Source: CAD feature listing. Evaluate the final solid. Frame: model axes, mm. A direction names the side the tool comes from. Give positions to 0.01 mm unless a question says otherwise; leave off trailing zeros. Loops run counter-clockwise (first coordinate to the right, second up) from the corner with the lowest first, then second, coordinate; pieces in that order, holes last. Notation, with made-up numbers: (51.5, 3.5) -> (56.5, 3.5) arc R32 ccw to (56.5, 39.5) -> close; hole circle Ø5 at (79, 36). An arc over 180 degrees is marked (long way). Answer as a JSON object with one key per item and string values. Group by question number.
from build123d import *

# Parameters (mm, degrees)
SKETCH_1_R          = 2.7000000000000006
SKETCH_1_R_2        = 2.700000000000003
EXTRUDE_1_DEPTH     = 5.1
SKETCH_2_R          = 4.999999999999998
SKETCH_2_R_2        = 2.5
EXTRUDE_2_DEPTH     = 5.94
CUT_EXTRUDE_1_DEPTH = 3.5
CUT_EXTRUDE_START   = -0.6
CUT_EXTRUDE_3_DEPTH = 0.6
EXTRUDE_START       = 1.2
SKETCH_6_R          = 4.999999999999998
SKETCH_6_R_2        = 2.5
SKETCH_6_R_3        = 5
SKETCH_6_R_4        = 2.4999999999999987
EXTRUDE_4_DEPTH     = 1.2
SKETCH_7_R          = 2.6000000000000005
CUT_EXTRUDE_4_DEPTH = 33.57721194023454
SKETCH_8_R          = 2.6
CUT_EXTRUDE_5_DEPTH = 31.8406734329677
SKETCH_10_R         = 2.7
CUT_EXTRUDE_6_DEPTH = 33.57721194023454
SKETCH_11_R         = 2.700000000000001
CUT_EXTRUDE_7_DEPTH = 31.8406734329677


with BuildPart() as part:
    # Эскиз1 → Бобышка-Вытянуть1 (new body)
    with BuildSketch(Plane(origin=(0, 0, 0), x_dir=(1, 0, 0), z_dir=(0, 1, 0))):
        with BuildLine():
            Line((6.718023264525762, 8.928267668376021), (7.161238337218641, 11.37785065819786))
            Line((7.161238337218641, 11.37785065819786), (7.294846288705666, 12.560700282216452))
            Line((7.294846288705666, 12.560700282216452), (7.085001061393901, 12.665407082864023))
            Line((7.085001061393901, 12.665407082864023), (6.15987792536569, 11.916319971156167))
            Line((6.15987792536569, 11.916319971156167), (5.853623131200735, 12.10383694173367))
            Line((5.853623131200735, 12.10383694173367), (5.855060736117009, 13.29420757772634))
            Line((5.855060736117009, 13.29420757772634), (5.634886528714601, 13.37496556136943))
            Line((5.634886528714601, 13.37496556136943), (4.798663389284832, 12.527784837542624))
            Line((4.798663389284832, 12.527784837542624), (4.473480547373511, 12.680135526842204))
            Line((4.473480547373511, 12.680135526842204), (4.342730025112913, 13.863304415323501))
            Line((4.342730025112913, 13.863304415323501), (4.114949999467502, 13.919114749889351))
            Line((4.114949999467502, 13.919114749889351), (3.3779694438823102, 12.984318526945106))
            Line((3.3779694438823102, 12.984318526945106), (3.0378804853992434, 13.099618628946285))
            Line((3.0378804853992434, 13.099618628946285), (2.776558986480811, 14.260952083189514))
            Line((2.776558986480811, 14.260952083189514), (2.54399037483231, 14.291124494483034))
            Line((2.54399037483231, 14.291124494483034), (1.9153675367628848, 13.280274532718662))
            Line((1.9153675367628848, 13.280274532718662), (1.56457875493138, 13.35709799101592))
            Line((1.56457875493138, 13.35709799101592), (1.175918359734634, 14.482232389631033))
            Line((1.175918359734634, 14.482232389631033), (0.9414376205823001, 14.486393698794194))
            Line((0.9414376205823001, 14.486393698794194), (0.4289474421954887, 13.411992407470256))
            Line((0.42894744219548875, 13.411992407470256), (0.07179746795026506, 13.449389053044667))
            Line((0.07179746795026506, 13.449389053044667), (-0.4393947883485354, 14.524408492330128))
            Line((-0.43939478834853546, 14.524408492330128), (-0.6728875469021285, 14.502507231398162))
            Line((-0.6728875469021285, 14.502507231398162), (-1.062906477097084, 13.377843036257644))
            Line((-1.062906477097084, 13.377843036257644), (-1.4220003362283888, 13.375350339371238))
            Line((-1.4220003362283888, 13.375350339371238), (-2.049401918098927, 14.386958748197415))
            Line((-2.049401918098927, 14.386958748197415), (-2.279018807507275, 14.33926579666565))
            Line((-2.279018807507275, 14.33926579666565), (-2.5417426516817105, 13.178248785832608))
            Line((-2.5417426516817105, 13.178248785832608), (-2.898339045786024, 13.13589757669542))
            Line((-2.898339045786024, 13.13589757669542), (-3.6341901158202092, 14.071583165165732))
            Line((-3.6341901158202092, 14.071583165165732), (-3.8570911851181764, 13.998688399693854))
            Line((-3.8570911851181764, 13.998688399693854), (-3.989270518385492, 12.815678280718325))
            Line((-3.989270518385492, 12.815678280718325), (-4.3389589867331635, 12.733992368173748))
            Line((-4.3389589867331635, 12.733992368173748), (-5.174158380979493, 13.582182376127184))
            Line((-5.174158380979493, 13.582182376127184), (-5.3875867419063175, 13.48498737481814))
            Line((-5.3875867419063175, 13.48498737481814), (-5.3875867419063175, 12.2946158707315))
            Line((-5.3875867419063175, 12.2946158707315), (-5.751610974482103, 12.12883970299033))
            Line((-5.751610974482103, 12.12883970299033), (-6.666748566138722, 12.905854249247858))
            Line((-6.666748566138722, 12.905854249247858), (-7.13096440438616, 12.63943472468846))
            Line((-7.13096440438616, 12.63943472468846), (-7.025830916712447, 12.175864106991055))
            ThreePointArc((-7.025830916712449, 12.175864106991055), (-10.264322646127633, 9.799709596012173), (-12.51111253150909, 6.470163958468902))
            Line((-12.51111253150909, 6.470163958468902), (-5.241071220187256, 3.924995297345621))
            Line((-5.241071220187256, 3.924995297345621), (-4.737733567637334, 1.5980865565051285))
            ThreePointArc((-4.737733567637334, 1.5980865565051288), (-4.061430338102922, -2.9162962141622684), (1.55e-15, -5))
            Line((2.2e-16, -5), (21.46693589645179, -5.388260461869603))
            ThreePointArc((21.46693589645179, -5.388260461869605), (26.46693589645179, -0.3882604618696045), (21.46693589645179, 4.611739538130397))
            Line((21.46693589645179, 4.611739538130397), (7.924308406385933, 7.062073595968816))
            ThreePointArc((7.924308406385932, 7.062073595968816), (7.00463576208043, 7.790569444059032), (6.718023264525762, 8.928267668376021))
        make_face()
        with Locations(Location((21.46693589645179, -0.3882604618696027, 0), (0, 0, 270))):
            Circle(SKETCH_1_R, mode=Mode.SUBTRACT)
        with Locations(Location((-2.22e-15, -1.39e-15, 0), (0, 0, 270))):
            Circle(SKETCH_1_R_2, mode=Mode.SUBTRACT)
    extrude(amount=EXTRUDE_1_DEPTH)

    # Эскиз2 → Бобышка-Вытянуть2 (add)
    with BuildSketch(Plane(origin=(0, 5.1, 0), x_dir=(1, 0, 0), z_dir=(0, 1, 0))):
        with Locations(Location((0, 0, 0), (0, 0, 270))):
            Circle(SKETCH_2_R)
        with Locations(Location((0, 0, 0), (0, 0, 270))):
            Circle(SKETCH_2_R_2, mode=Mode.SUBTRACT)
    extrude(amount=EXTRUDE_2_DEPTH)

    # Эскиз4 → Вырез-Вытянуть1 (cut)
    with BuildSketch(Plane.XZ):
        with BuildLine():
            Line((-5.241071220187255, -3.924995297345621), (-7.025830916712447, -12.175864106991055))
            ThreePointArc((-7.025830916712447, -12.175864106991055), (-10.264322646127628, -9.799709596012166), (-12.511112531509088, -6.470163958468901))
            Line((-12.511112531509088, -6.470163958468901), (-5.241071220187255, -3.924995297345621))
        make_face()
    extrude(amount=-CUT_EXTRUDE_1_DEPTH, mode=Mode.SUBTRACT)

    # Эскиз5 → Вырез-Вытянуть3 (cut)
    with BuildSketch(Plane(origin=(0, 5.1, 0), x_dir=(1, 0, 0), z_dir=(0, 1, 0)).offset(CUT_EXTRUDE_START)):
        with BuildLine():
            Line((-5.241071220187255, 3.924995297345621), (-7.025830916712447, 12.175864106991055))
            ThreePointArc((-7.025830916712447, 12.175864106991055), (-10.264322646127628, 9.799709596012168), (-12.511112531509088, 6.470163958468901))
            Line((-12.511112531509088, 6.470163958468901), (-5.241071220187255, 3.924995297345621))
        make_face()
    extrude(amount=CUT_EXTRUDE_3_DEPTH, mode=Mode.SUBTRACT)

    # Эскиз6 → Бобышка-Вытянуть4 (add)
    # profile 1 of 2: a face of its own
    with BuildSketch(Plane.XZ.offset(EXTRUDE_START)):
        with Locations(Location((0, 0, 0), (0, 0, 270))):
            Circle(SKETCH_6_R)
        with Locations(Location((0, 0, 0), (0, 0, 90))):
            Circle(SKETCH_6_R_2, mode=Mode.SUBTRACT)
    # profile 2 of 2: a face of its own
    with BuildSketch(Plane.XZ.offset(EXTRUDE_START)):
        with Locations(Location((21.46693589645179, 0.38826046186960295, 0), (0, 0, 270))):
            Circle(SKETCH_6_R_3)
        with Locations(Location((21.46693589645179, 0.38826046186960295, 0), (0, 0, 270))):
            Circle(SKETCH_6_R_4, mode=Mode.SUBTRACT)
    extrude(amount=-EXTRUDE_4_DEPTH)

    # Эскиз7 → Вырез-Вытянуть4 (cut, through all)
    with BuildSketch(Plane(origin=(0, 11.04, 0), x_dir=(1, 0, 0), z_dir=(0, 1, 0))):
        with Locations(Location((0, 0, 0), (0, 0, 270))):
            Circle(SKETCH_7_R)
    extrude(amount=-CUT_EXTRUDE_4_DEPTH, mode=Mode.SUBTRACT)

    # Эскиз8 → Вырез-Вытянуть5 (cut, through all)
    with BuildSketch(Plane(origin=(0, 5.1, 0), x_dir=(1, 0, 0), z_dir=(0, 1, 0))):
        with Locations(Location((21.46693589645179, -0.38826046186960295, 0), (0, 0, 270))):
            Circle(SKETCH_8_R)
    extrude(amount=-CUT_EXTRUDE_5_DEPTH, mode=Mode.SUBTRACT)

    # Эскиз10 → Вырез-Вытянуть6 (cut, through all)
    with BuildSketch(Plane(origin=(0, 11.04, 0), x_dir=(1, 0, 0), z_dir=(0, 1, 0))):
        with Locations(Location((0, 0, 0), (0, 0, 270))):
            Circle(SKETCH_10_R)
    extrude(amount=-CUT_EXTRUDE_6_DEPTH, mode=Mode.SUBTRACT)

    # Эскиз11 → Вырез-Вытянуть7 (cut, through all)
    with BuildSketch(Plane(origin=(0, 5.1, 0), x_dir=(1, 0, 0), z_dir=(0, 1, 0))):
        with Locations(Location((21.46693589645179, -0.38826046186960295, 0), (0, 0, 270))):
            Circle(SKETCH_11_R)
    extrude(amount=-CUT_EXTRUDE_7_DEPTH, mode=Mode.SUBTRACT)


solid = part.part
(1) Section query B-B on y = 6.5. Return the cut outline in (x, z).
(2) First-contact query: pin 1 (5 mm diameter, centred on x = 9, z = -10.5, fed in from +Y); pin 2 (2 mm diameter, centred on x = 6.5, z = -6, fed in from -Y); pin 3 (1.3 mm diameter, centred on y = 2, z = -13, fed in from -X). Flat tips, straight axial feed; report the tip coordinate or a pass-through.
(3) Material intervals for line 1 (X direction, y = 7.2, z = 0); line 2 (X direction, y = -0.75, z = 0) (3 decimals); line 3 (Y direction, x = 18.5, z = -2.75), sorted ascending. Write a range as from..to.
(4) Section query C-C on z = -5.75. Return the cut outline in (x, y), plus the area to 3 significant figures.
(5) Access query for faces 1 (the face through (5.223, 2.514, -12.957)), 2 (the face through (6.937, 2.514, -10.136)), 3 (the face through (-9, 3.5, -8)). Directions: +Z, -Z, +X, -X, +Y, -Y. A direction counts if a zero-diameter tool reaches every point of the face in a straight line with its end or side. Return the directions, or none.
(6) Section query D-D on x = 17.5. Return the cut outline in (y, z), plus the area to 3 significant figures.
(7) Mould query, pull axis Z, two halves, no side actions, for faces 4 (the face through (-2.2, 11.04, 2.2)), 5 (the face through (-0.18, 2.51, -13.98)), 6 (the face through (7, 2.5, -7.8)). Classes: pulls with the +Z half, pulls with the -Z half, needs draft (parallel to the pull), parting line crosses it, or undercut.
Result:
{
 "1": {"outline": "circle Ø10 at (0, 0); hole circle Ø5.4 at (0, 0)"},
 "2": {"pin 1": "y = 5.1", "pin 2": "y = 0", "pin 3": "x = -7.13"},
 "3": {"line 1": "-5..-2.7, 2.7..5", "line 2": "-5..-2.7, 2.7..5, 16.482..18.795, 24.139..26.452", "line 3": "-1.2..5.1"},
 "4": {"outline": "(-10.45, 3.5) -> (-5.64, 3.5) -> (-5.64, 0) -> (15.18, 0) -> (15.18, 5.1) -> (-5.64, 5.1) -> (-5.64, 4.5) -> (-10.45, 4.5) -> close", "area": "111 mm²"},
 "5": {"face 1": "-Z, +Y, -Y", "face 2": "+X, +Y, -Y", "face 3": "+Z, -X, -Y"},
 "6": {"outline": "(-1.2, -2.66) -> (0, -2.66) -> (0, -5.33) -> (5.1, -5.33) -> (5.1, 5.32) -> (0, 5.32) -> (0, 3.43) -> (-1.2, 3.43) -> close", "area": "61.6 mm²"},
 "7": {"face 4": "needs draft", "face 5": "pulls with the -Z half", "face 6": "undercut"}
}
